from build123d import *

# Parameters (mm, degrees)
BOSS_EXTRUDE1_DEPTH = 20
FILLET1_R           = 2.5
FILLET2_R           = 1


with BuildPart() as part:
    # Sketch1 → Boss-Extrude1 (new body)
    with BuildSketch(Plane(origin=(0, 0, 0), x_dir=(1, 0, 0), z_dir=(0, 1, 0))):
        with BuildLine():
            Line((36.117717004, 19.916765755), (36.117717004, 0))
            Line((36.117717004, 0), (11.2960761, 0))
            Line((11.2960761, 0), (11.2960761, 125))
            Line((11.2960761, 125), (36.984740388, 125))
            Line((36.984740388, 125), (36.984740388, 99.311335711))
            Line((36.984740388, 99.311335711), (36.117717004, 76.198969481))
            add(Edge.make_bspline(
                [(36.117717004, 76.198969481), (37.079035526, 78.513840699), (37.821716785, 81.825002834), (39.841285118, 85.425058127), (41.21525815, 87.372030125), (42.770642161, 89.163856041), (44.531204538, 90.74523712), (46.455711817, 92.116095649), (48.524028366, 93.283848821), (50.743017021, 94.262315505), (53.129690053, 95.000321934), (56.595091524, 95.697992737), (59.296350256, 95.909848431), (61.137534681, 95.892786365)],
                knots=[0, 0, 0, 0, 0.21768002, 0.286847597, 0.354813327, 0.422943008, 0.491013117, 0.558398108, 0.626322787, 0.695519685, 0.767143763, 0.841303709, 1, 1, 1, 1], degree=3))
            add(Edge.make_bspline(
                [(61.137534681, 95.892786365), (63.395086057, 95.903685841), (66.735821106, 95.621334637), (70.981289729, 94.544167423), (73.935977914, 93.451744493), (76.70594677, 92.030063316), (79.28991441, 90.280281683), (81.71457152, 88.236417621), (83.926657745, 85.882399021), (85.942182726, 83.286794391), (87.670170765, 80.442277233), (89.170620742, 77.406405656), (90.390921152, 74.14710145), (91.289056083, 70.663202505), (92.199939451, 65.644798855), (92.480055787, 61.741506128), (92.449464923, 59.081450654)],
                knots=[0, 0, 0, 0, 0.12448834, 0.183662525, 0.240987058, 0.297785083, 0.354848785, 0.412664579, 0.472231373, 0.532594602, 0.593487538, 0.655372754, 0.719036994, 0.784951013, 0.85343042, 1, 1, 1, 1], degree=3))
            Line((92.449464923, 59.081450654), (92.449464923, 35.102061038))
            add(Edge.make_bspline(
                [(92.449464923, 35.102061038), (92.481706946, 32.417206566), (92.200218527, 28.481210749), (91.291825145, 23.429095843), (90.392084489, 19.936614782), (89.162904767, 16.673762861), (87.685043138, 13.625497661), (85.932163927, 10.795769529), (83.93534446, 8.202568905), (81.712640064, 5.873123122), (79.290226272, 3.851331714), (76.698739641, 2.131042563), (73.936325888, 0.70776156), (70.984961829, -0.392480025), (66.728426656, -1.4160417), (63.397954668, -1.731864559), (61.137534681, -1.709274673)],
                knots=[0, 0, 0, 0, 0.147807026, 0.216676018, 0.282534324, 0.346144753, 0.408386101, 0.468840468, 0.529152677, 0.588339784, 0.645814146, 0.702576919, 0.759326937, 0.816603017, 0.875616881, 1, 1, 1, 1], degree=3))
            add(Edge.make_bspline(
                [(61.137534681, -1.709274673), (59.296350246, -1.726336751), (56.595091542, -1.514481022), (53.129690028, -0.816810273), (50.743017111, -0.078803702), (48.524028045, 0.899662475), (46.455712988, 2.067417488), (44.531200185, 3.438269202), (42.7706586, 5.019675936), (41.215196821, 6.811405891), (39.841515083, 8.758737328), (38.654148229, 10.871953586), (37.24125462, 14.565590682), (36.509346228, 17.63130127), (36.117717004, 19.916765755)],
                knots=[0, 0, 0, 0, 0.150649959, 0.221049795, 0.289042338, 0.354730766, 0.41921148, 0.483179869, 0.547798639, 0.612473961, 0.676993644, 0.742654238, 0.810316636, 1, 1, 1, 1], degree=3))
        make_face()
        with BuildLine():
            Line((66.785572731, 35.969084423), (66.785572731, 58.214427269))
            add(Edge.make_bspline(
                [(66.785572731, 58.214427269), (66.771829802, 60.406770749), (66.417836342, 63.625724633), (64.723817468, 67.39558891), (63.000354868, 69.655005362), (60.827701936, 71.453642984), (57.173659281, 73.229809674), (54.023085733, 73.637658685), (51.872770511, 73.622671423)],
                knots=[0, 0, 0, 0, 0.271016724, 0.390594505, 0.504399399, 0.61771336, 0.734495657, 1, 1, 1, 1], degree=3))
            add(Edge.make_bspline(
                [(51.872770511, 73.622671423), (49.759720525, 73.644159543), (46.659201079, 73.209984567), (43.036444514, 71.44905498), (40.849183836, 69.648312437), (39.063540587, 67.412914524), (37.394409246, 63.61564329), (36.967690872, 60.41840948), (36.984740388, 58.214427269)],
                knots=[0, 0, 0, 0, 0.261213344, 0.378316389, 0.492729113, 0.608095085, 0.728001293, 1, 1, 1, 1], degree=3))
            Line((36.984740388, 58.214427269), (36.984740388, 35.969084423))
            add(Edge.make_bspline(
                [(36.984740388, 35.969084423), (36.967648998, 33.758379722), (37.387401392, 30.548144965), (39.070893069, 26.743120106), (40.841102205, 24.488680021), (43.031159697, 22.68091473), (46.671799289, 20.967376381), (49.754651115, 20.503707396), (51.872770511, 20.536068173)],
                knots=[0, 0, 0, 0, 0.272641397, 0.39238352, 0.508393071, 0.622649228, 0.739144111, 1, 1, 1, 1], degree=3))
            add(Edge.make_bspline(
                [(51.872770511, 20.536068173), (54.028327267, 20.509831436), (57.160874782, 20.947979289), (60.832954812, 22.676374312), (63.008458872, 24.482146365), (64.716399441, 26.760301899), (66.424893748, 30.538107854), (66.771576456, 33.77007391), (66.785572731, 35.969084423)],
                knots=[0, 0, 0, 0, 0.265139708, 0.381314935, 0.494473274, 0.608929805, 0.728343363, 1, 1, 1, 1], degree=3))
        make_face(mode=Mode.SUBTRACT)
    extrude(amount=-BOSS_EXTRUDE1_DEPTH)

    # Fillet1
    fillet1_edges = [part.edges().sort_by_distance(p)[0] for p in [
        (36.117717004, -10, -76.198969481),
        (36.117717004, -10, -19.916765755),
    ]]
    fillet(fillet1_edges, radius=FILLET1_R)

    # Fillet2
    fillet2_edges = [part.edges().sort_by_distance(p)[0] for p in [
        (36.117717004, -10, 0),
        (11.2960761, -10, 0),
        (11.2960761, -10, -125),
        (36.984740388, -10, -125),
    ]]
    fillet(fillet2_edges, radius=FILLET2_R)


solid = part.part
Part model, mm, in its own coordinate system. A direction names the side the tool comes from. Give positions to 0.01 mm unless a question says otherwise; leave off trailing zeros. Loops run counter-clockwise (first coordinate to the right, second up) from the corner with the lowest first, then second, coordinate; pieces in that order, holes last. Notation, with made-up numbers: M 36.5,-33 L 47.5,-33 A18 cw 47.5,2 Z; hole C 35.25,15.5 d11. An arc over 180 degrees is marked long. Put each result on its own line as item: value. Start each with the question number.
1) Saw through at A-A (z = -47). List the corners of the cut face in (x, y), then the cut area to 3 significant figures.
2) Saw through at B-B (z = -116). List the corners of the cut face in (x, y).
3) Probe probe 1 along Z at (x, y) = (18, -12); probe 2 along X at (y, z) = (-15.5, -115); probe 3 along X at (y, z) = (-10.75, -87). List the from-to ranges inside material, lowest first.
4) Flat gauge pins, fed straight in: pin 1 (6 mm diameter, centred on y = -8.5, z = -50, fed in from +X); pin 2 (3 mm diameter, centred on x = 62.5, y = -14, fed in from -Z); pin 3 (12 mm diameter, centred on x = 45.5, y = -12.5, fed in from +Z); pin 4 (10 mm diameter, centred on x = 65.5, z = -45, fed in from -Y). Where does each tip first touch, or does it go through?
5) 3-axis set-ups, long thin cutter, end or side, ignore diameter. For faces 1 (the flat face through (36.985, -10, -112)), 2 (the flat face through (36.985, -10, -47)), 3 (the flat face through (36.118, -10, -4)), 4 (the flat face through (24, -10, 0)): which of +Z, -Z, +X, -X, +Y, -Y reach the whole face in a straight line?
Numbers:
1. outline: M 11.3,-20 L 36.98,-20 L 36.98,0 L 11.3,0 Z; M 66.79,-20 L 92.45,-20 L 92.45,0 L 66.79,0 Z
1. area: 1,030 mm^2
2. outline: M 11.3,-20 L 36.98,-20 L 36.98,0 L 11.3,0 Z
3. probe 1: -125 to 0
3. probe 2: 11.3 to 36.98
3. probe 3: 11.3 to 37.2, 40.97 to 82.86
4. pin 1: x = 92.45
4. pin 2: z = -95.89
4. pin 3: z = 0.3
4. pin 4: y = -20
5. face 1: -Z, +X, +Y, -Y
5. face 2: +Y, -Y
5. face 3: +Z, +Y, -Y
5. face 4: +Z, -X, +Y, -Y
